Source: CAD feature listing. Evaluate the final solid. Frame: model axes, mm. Face numbers are marked on the shaded views. A direction names the side the tool comes from. Give positions to 0.01 mm unless a question says otherwise; leave off trailing zeros. Loops run counter-clockwise (first coordinate to the right, second up) from the corner with the lowest first, then second, coordinate; pieces in that order, holes last.
from build123d import *

# Parameters (mm, degrees)
SKETCH1_W                                         = 35
SKETCH1_H                                         = 30
BOSS_EXTRUDE1_DEPTH                               = 3
SKETCH2_W                                         = 35
SKETCH2_H                                         = 30
SKETCH2_W_2                                       = 29
SKETCH2_H_2                                       = 24
BOSS_EXTRUDE2_DEPTH                               = 3
SKETCH3_W                                         = 10
SKETCH3_H                                         = 10
CUT_EXTRUDE1_DEPTH                                = 3
CSK_FOR_M2_5_FLAT_HEAD_MACHINE_SCREW1_D           = 2.9
CSK_FOR_M2_5_FLAT_HEAD_MACHINE_SCREW1_DEPTH       = 5
CSK_FOR_M2_5_FLAT_HEAD_MACHINE_SCREW1_CSINK_D     = 5.5
CSK_FOR_M2_5_FLAT_HEAD_MACHINE_SCREW1_CSINK_ANGLE = 90
CSK_FOR_M2_5_FLAT_HEAD_MACHINE_SCREW1_TIP         = 0.871247898
BOSS_EXTRUDE4_DEPTH                               = 3
FILLET1_R                                         = 1
BOSS_EXTRUDE5_REACH                               = 26.494
SKETCH15_W                                        = 29
SKETCH15_H                                        = 3
SKETCH16_W                                        = 29
SKETCH16_H                                        = 3
CUT_EXTRUDE6_DEPTH                                = 3
FILLET2_R                                         = 4
FILLET3_R                                         = 2
SKETCH21_W                                        = 14.289809421
SKETCH21_H                                        = 25
BOSS_EXTRUDE7_DEPTH                               = 3
SKETCH23_W                                        = 32
SKETCH23_H                                        = 6
BOSS_EXTRUDE8_DEPTH                               = 3
BOSS_EXTRUDE10_DEPTH                              = 32
SKETCH30_R                                        = 1.25
CUT_EXTRUDE13_DEPTH                               = 56.03815634
SKETCH32_R                                        = 4.5
SKETCH32_R_2                                      = 2.4
BOSS_EXTRUDE12_DEPTH                              = 5
SKETCH33_R                                        = 2.75
CUT_EXTRUDE15_DEPTH                               = 4.5
SKETCH32_4_R                                      = 2.4
SKETCH32_4_R_2                                    = 1.25
BOSS_EXTRUDE13_DEPTH                              = 3
SKETCH34_R                                        = 2.75
CUT_EXTRUDE17_DEPTH                               = 4.5
CUT_EXTRUDE18_DEPTH                               = 54.18081095


with BuildPart() as part:
    # Sketch1 → Boss-Extrude1 (new body)
    with BuildSketch(Plane.XY):
        Rectangle(SKETCH1_W, SKETCH1_H)
    extrude(amount=-BOSS_EXTRUDE1_DEPTH)

    # Sketch2 → Boss-Extrude2 (add)
    with BuildSketch(Plane(origin=(0, 0, -3), x_dir=(-1, 0, 0), z_dir=(0, 0, -1))):
        Rectangle(SKETCH2_W, SKETCH2_H)
        Rectangle(SKETCH2_W_2, SKETCH2_H_2, mode=Mode.SUBTRACT)
    extrude(amount=BOSS_EXTRUDE2_DEPTH)

    # Sketch3 → Cut-Extrude1 (cut)
    with BuildSketch(Plane.XY):
        with Locations((0, -4.5)):
            Rectangle(SKETCH3_W, SKETCH3_H)
    extrude(amount=-CUT_EXTRUDE1_DEPTH, mode=Mode.SUBTRACT)

    # CSK for M2.5 Flat Head Machine Screw1
    with Locations(Plane.XY):
        with Locations((10.5, 8), (-10.5, -4.5), (-10.5, 8), (10.5, -4.5)):
            CounterSinkHole(CSK_FOR_M2_5_FLAT_HEAD_MACHINE_SCREW1_D / 2, CSK_FOR_M2_5_FLAT_HEAD_MACHINE_SCREW1_CSINK_D / 2, depth=CSK_FOR_M2_5_FLAT_HEAD_MACHINE_SCREW1_DEPTH, counter_sink_angle=CSK_FOR_M2_5_FLAT_HEAD_MACHINE_SCREW1_CSINK_ANGLE)
            with Locations((0, 0, -(CSK_FOR_M2_5_FLAT_HEAD_MACHINE_SCREW1_DEPTH + CSK_FOR_M2_5_FLAT_HEAD_MACHINE_SCREW1_TIP / 2))):  # 118° drill point
                Cone(0, CSK_FOR_M2_5_FLAT_HEAD_MACHINE_SCREW1_D / 2, CSK_FOR_M2_5_FLAT_HEAD_MACHINE_SCREW1_TIP, mode=Mode.SUBTRACT)

    # Sketch11 → Boss-Extrude4 (add)
    with BuildSketch(Plane.ZY.offset(17.5)):
        Polygon((-6, 15), (-9, 15), (-14.289809421, -15), (-6, -15), align=None)
    boss_extrude4 = extrude(amount=-BOSS_EXTRUDE4_DEPTH)

    # Mirror1: Boss-Extrude4 across plane
    add(boss_extrude4.mirror(Plane(origin=(0, 0, 0), x_dir=(0, 0, 1), z_dir=(1, 0, 0))))

    # Fillet1
    fillet1_edges = [part.edges().sort_by_distance(p)[0] for p in [
        (5, 0.5, -1.5),
        (5, -9.5, -1.5),
        (-5, -9.5, -1.5),
        (-5, 0.5, -1.5),
    ]]
    fillet(fillet1_edges, radius=FILLET1_R)

    # Boss-Extrude5: up to this face of the body (flat: up to its plane)
    boss_extrude5_end = Plane(part.part.faces().sort_by_distance((16, 0, -11.644904711))[0])
    # Sketch15 → Boss-Extrude5 (add, up to the picked face)
    with BuildSketch(Plane(origin=(0, 0, -6), x_dir=(-1, 0, 0), z_dir=(0, 0, -1)), mode=Mode.PRIVATE) as boss_extrude5_sk1:
        with Locations((0, 13.5)):
            Rectangle(SKETCH15_W, SKETCH15_H)
    boss_extrude5_tool1 = split(extrude(boss_extrude5_sk1.sketch, amount=BOSS_EXTRUDE5_REACH, mode=Mode.PRIVATE), bisect_by=boss_extrude5_end, keep=Keep.BOTH, mode=Mode.PRIVATE)
    add(boss_extrude5_tool1.solids().sort_by(Axis((0, 13.5, -6), (0, 0, -1)))[0])

    # Sketch16 → Cut-Extrude6 (cut)
    with BuildSketch(Plane.XZ.offset(15)):
        with Locations((0, -4.5)):
            Rectangle(SKETCH16_W, SKETCH16_H)
    extrude(amount=-CUT_EXTRUDE6_DEPTH, mode=Mode.SUBTRACT)

    # Fillet2
    fillet2_edges = [part.edges().sort_by_distance(p)[0] for p in [
        (-17.5, 15, -4.5),
        (17.5, 15, -4.5),
    ]]
    fillet(fillet2_edges, radius=FILLET2_R)

    # Fillet3
    fillet3_edges = [part.edges().sort_by_distance(p)[0] for p in [
        (-14.5, 12, -6.264490471),
        (14.5, 12, -6.264490471),
    ]]
    fillet(fillet3_edges, radius=FILLET3_R)

    # Sketch21 → Boss-Extrude7 (add)
    with BuildSketch(Plane.ZY.offset(17.5)):
        with Locations((-7.144904711, -27.5)):
            Rectangle(SKETCH21_W, SKETCH21_H)
    extrude(amount=-BOSS_EXTRUDE7_DEPTH)

    # Sketch23 → Boss-Extrude8 (add)
    with BuildSketch(Plane.XY):
        with Locations((1.5, -18)):
            Rectangle(SKETCH23_W, SKETCH23_H)
    extrude(amount=-BOSS_EXTRUDE8_DEPTH)

    # Sketch27 → Boss-Extrude10 (add)
    with BuildSketch(Plane(origin=(17.5, 0, 0), x_dir=(0, 0, -1), z_dir=(1, 0, 0))):
        Polygon((3, -21), (3, -15.803847577), (6, -21), align=None)
    extrude(amount=-BOSS_EXTRUDE10_DEPTH)

    # Sketch30 → Cut-Extrude13 (cut, through all)
    with BuildSketch(Plane.ZY.offset(17.5)):
        with Locations((-7.144904711, -34)):
            Circle(SKETCH30_R)
    extrude(amount=-CUT_EXTRUDE13_DEPTH, mode=Mode.SUBTRACT)

    # Sketch32 → Boss-Extrude12 (add)
    with BuildSketch(Plane(origin=(-14.5, 0, 0), x_dir=(0, 0, -1), z_dir=(1, 0, 0))):
        with Locations((7.144904711, -34)):
            Circle(SKETCH32_R)
        with Locations(Location((7.144904711, -34, 0), (0, 0, 90))):
            Circle(SKETCH32_R_2, mode=Mode.SUBTRACT)
    extrude(amount=BOSS_EXTRUDE12_DEPTH)

    # Sketch33 → Cut-Extrude15 (cut)
    with BuildSketch(Plane.ZY.offset(17.5)):
        with Locations((-7.144904711, -34)):
            Circle(SKETCH33_R)
    extrude(amount=-CUT_EXTRUDE15_DEPTH, mode=Mode.SUBTRACT)

    # Sketch32<4> → Boss-Extrude13 (add)
    with BuildSketch(Plane(origin=(-14.5, 0, 0), x_dir=(0, 0, -1), z_dir=(1, 0, 0))):
        with Locations((7.144904711, -34)):
            Circle(SKETCH32_4_R)
        with Locations((7.144904711, -34)):
            Circle(SKETCH32_4_R_2, mode=Mode.SUBTRACT)
    extrude(amount=BOSS_EXTRUDE13_DEPTH)

    # Sketch34 → Cut-Extrude17 (cut)
    with BuildSketch(Plane.ZY.offset(17.5)):
        with Locations((-7.144904711, -34)):
            Circle(SKETCH34_R)
    extrude(amount=-CUT_EXTRUDE17_DEPTH, mode=Mode.SUBTRACT)

    # Sketch35 → Cut-Extrude18 (cut, through all)
    with BuildSketch(Plane(origin=(-14.5, 0, 0), x_dir=(0, 0, -1), z_dir=(1, 0, 0))):
        with BuildLine():
            Line((2.806290635, -35.194331572), (0, -25))
            Line((0, -25), (0, -40))
            Line((0, -40), (14.289809421, -40))
            Line((14.289809421, -40), (14.289809421, -25))
            Line((14.289809421, -25), (11.483518786, -35.194331572))
            ThreePointArc((11.483518786, -35.194331572), (7.144904711, -38.5), (2.806290635, -35.194331572))
        make_face()
    extrude(amount=-CUT_EXTRUDE18_DEPTH, mode=Mode.SUBTRACT)


solid = part.part
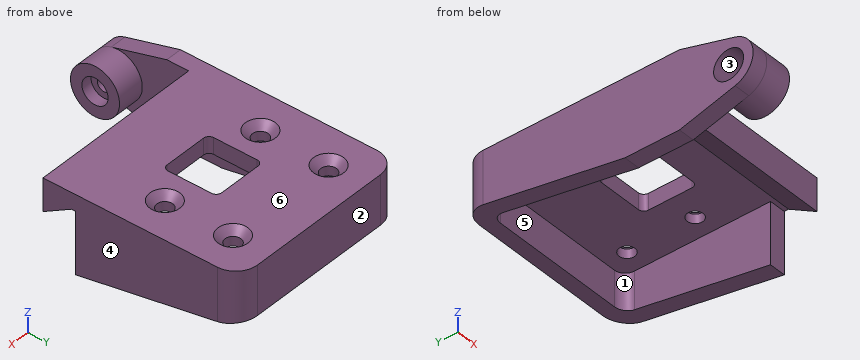
1) Pull-direction query (X, two-part tool) for the marked faces 4, 5 and 6; classes: released by +X, released by -X, zero draft, split by the parting line, or undercut.
Checks:
face 4: released by +X
face 5: undercut
face 6: zero draft
2) Contact query for flat-ended pins moving along their axis: P1, Ø8, axis at x = 9, z = -12.5, coming from the -Y side; P2, Ø8.5, axis at x = 5.5, y = -0.5, coming from the -Z side; P3, Ø2.5, axis at x = 0, z = -2, coming from the -Y side. Output: stop coordinate, or through.
Checks:
P1: stops at y = 12
P2: stops at z = -3
P3: stops at y = -21
3) Cut plane B-B (x = 0.5). Return loops of the section in (y, z).
Checks:
outline: (-21, -6) - (-15.8, -3) - (-9.5, -3) - (-9.5, 0) - (-21, 0) - close; (0.5, -3) - (12, -3) - (12, -9.53) - (15, -9) - (15, 0) - (0.5, 0) - close
4) Ray query, probe 1 along Y at (x, z) = (10.5, -1.8); probe 2 along X at (y, z) = (8, -2.4); probe 3 along X at (y, z) = (-1.5, -2.75). Return the intervals inside material, ascending.
Checks:
probe 1: y = -21 to -5.95, -3.05 to 6.55, 9.45 to 15
probe 2: x = -17.5 to -11.95, -9.05 to 9.05, 11.95 to 17.5
probe 3: x = -17.5 to -5, 5 to 17.5
5) Cut plane D-D (z = -12.75). Return loops of the section in (x, y), and give its area (3 significant figures).
Checks:
outline: (-17.5, -30.59) - (-14.5, -30.59) - (-14.5, -6.27) - (-17.5, -6.27) - close; (14.5, -15) - (17.5, -15) - (17.5, -6.27) - (14.5, -6.27) - close
area: 99.2 mm2
6) Cut plane A-A (x = 10.5). Return loops of the section in (y, z), and give its area (3 significant figures).
Checks:
outline: (-21, -6) - (-15.8, -3) - (-5.95, -3) - (-5.95, -1.3) - (-7.25, 0) - (-21, 0) - close; (-3.05, -3) - (6.55, -3) - (6.55, -1.3) - (5.25, 0) - (-1.75, 0) - (-3.05, -1.3) - close; (9.45, -3) - (12, -3) - (12, -9.53) - (15, -9) - (15, 0) - (10.75, 0) - (9.45, -1.3) - close
area: 114 mm2
7) Reachability of the marked faces 1, 2 and 3 from +Z, -Z, +X, -X, +Y, -Y: full face, straight path, thin tool, end or side. Return the list, or none.
Checks:
face 1: -Z
face 2: +Z, -Z, +X, -X, +Y
face 3: -X
8) Cut plane C-C (y = -4.5). Return loops of the section in (x, z).
Checks:
outline: (-17.5, -12.44) - (-14.5, -12.44) - (-14.5, -3) - (-11.95, -3) - (-11.95, -1.3) - (-13.25, 0) - (-17.5, 0) - close; (-9.05, -3) - (-5, -3) - (-5, 0) - (-7.75, 0) - (-9.05, -1.3) - close; (5, -3) - (9.05, -3) - (9.05, -1.3) - (7.75, 0) - (5, 0) - close; (11.95, -3) - (14.5, -3) - (14.5, -12.44) - (17.5, -12.44) - (17.5, 0) - (13.25, 0) - (11.95, -1.3) - close
